Check sheet for the modelled part. Datum: model origin and axes. Units: mm. Face numbers are marked on the shaded views. A direction names the side the tool comes from. Give positions to 0.01 mm unless a question says otherwise; leave off trailing zeros. Write each loop counter-clockwise with the first axis right and the second up, starting at its lowest first coordinate (ties: lowest second). Pieces come first, ordered by that corner, then holes. Notation, with made-up numbers: M -24,-23.75 L -13,-23.75 A10 cw -13,-6.75 Z; hole C -34.5,54.25 d11. An arc over 180 degrees is marked long. Use CSV: the item, a comma, the result in double quotes. Start each with the question number.
1. Cross-section at B-B, the plane z = 12.5. Enter the section's corners in (x, y).
2. Depth check by flat-ended pin: P1, Ø5, axis at x = 1, y = 0.5, coming from the -Z side; P2, Ø1.5, axis at y = -6, z = 6, coming from the -X side; P3, Ø1, axis at y = -3.5, z = 5.5, coming from the -X side. Enter the tip coordinate at first touch or a pass-through.
3. Cross-section at A-A, the plane x = 0. Enter the section's corners in (y, z).
4. Scan lines: line 1 (Y direction, x = 0, z = 5); line 2 (X direction, y = -0.5, z = 3.25); line 3 (X direction, y = 0.25, z = 12). Record each from-to range of solid material in increasing order.
5. Access from +Z, -Z, +X, -X, +Y, -Y to the whole of each face (thin tool, end or side, straight path). Record for the marked faces 4 and 5.
6. Cross-section at C-C, the plane z = 5.25. Enter the section's corners in (x, y).
7. Mould release check, pull along X, two halves, no side actions. Record for the marked faces 1, 2 and 3: +X half, -X half, draft (parallel to the pull), parting line (faces both ways), or undercut.
Autodesk Inventor part; units mm, degrees
ref_plane "YZ Plane" through (0, 0, 0) normal (1, 0, 0) x (0, 1, 0)
ref_plane "XZ Plane" through (0, 0, 0) normal (0, 1, 0) x (-1, 0, 0)
ref_plane "XY Plane" through (0, 0, 0) normal (0, 0, 1) x (1, 0, 0)
sketch "Skizze1" plane through (0, 0, 0) normal (0, 0, 1) x (1, 0, 0)
  circle A0 centre (0, 0) radius 8.5
  dimension "d0" = 17
extrude "Extrusion1" add sketch "Skizze1" along normal blind 19
fillet "Rundung1" radius 2 2 edges at (-8.5, 0, 19) (-8.5, 0, 0)
sketch "Skizze2" plane through (0, 0, 19) normal (0, 0, 1) x (1, 0, 0)
  arc A0 (-4.1, 0) -> (4.1, 0) centre (0, 0) ccw
  line L0 (-4.1, 0) -> (4.1, 0)
  dimension "d4" = 8.2
extrude "Extrusion2" cut sketch "Skizze2" against normal blind 8.2
sketch "Skizze3" plane through (0, 0, 0) normal (0, 0, -1) x (-1, 0, 0)
  arc A0 (1.462, -2.15) -> (-1.462, -2.15) centre (0, 0) ccw
  line L0 (-1.462, -2.15) -> (1.462, -2.15)
  point P0 (0, -2.15)
  dimension "d8" = 5.2
extrude "Extrusion3" cut sketch "Skizze3" against normal blind 8.2
properties part number "Connector 001"
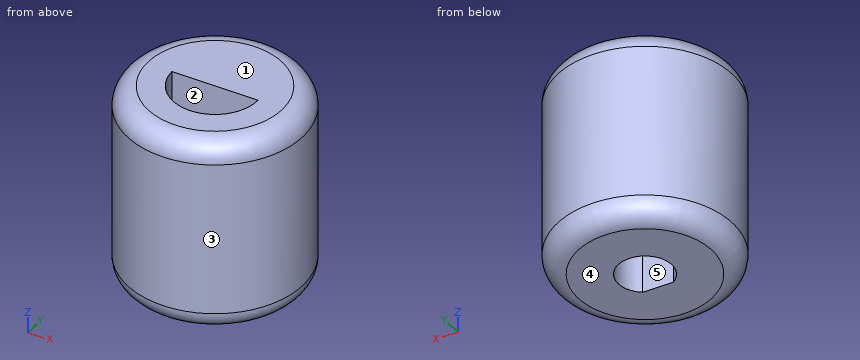
Worked answers:
1,outline,"C 0,0 d17; hole M -4.1,0 A4.1 ccw 4.1,0 Z"
2,P1,"stops at z = 0"
2,P2,"stops at x = -6.68"
2,P3,"stops at x = -7.95"
3,outline,"M -8.5,2 A2 ccw -6.5,0 L -2.15,0 L -2.15,8.2 L 2.6,8.2 L 2.6,0 L 6.5,0 A2 ccw 8.5,2 L 8.5,17 A2 ccw 6.5,19 L 0,19 L 0,10.8 L -4.1,10.8 L -4.1,19 L -6.5,19 A2 ccw -8.5,17 Z"
4,line 1,"y = -8.5 to -2.15, 2.6 to 8.5"
4,line 2,"x = -8.49 to -2.55, 2.55 to 8.49"
4,line 3,"x = -8.5 to 8.5"
5,face 4,"-Z, +X, -X, +Y, -Y"
5,face 5,"-Z"
6,outline,"C 0,0 d17; hole M -1.46,-2.15 L 1.46,-2.15 A2.6 ccw long Z"
7,face 1,"draft"
7,face 2,"undercut"
7,face 3,"parting line"
